Geometry: final body of the model. Coordinates: model frame, mm. Face numbers are marked on the shaded views. A direction names the side the tool comes from. Give positions to 0.01 mm unless a question says otherwise; leave off trailing zeros. Loops run counter-clockwise (first coordinate to the right, second up) from the corner with the lowest first, then second, coordinate; pieces in that order, holes last.
1. Draft query along X for the marked faces 3, 4 and 5. Return one class per face: +X half, -X half, draft (parallel to the pull), parting line (faces both ways), or undercut.
2. Section A-A, the plane y = 0. State how many separate pieces and enclosed holes the cut face has, then the cut area to 4 significant figures.
3. First-contact query: P1, Ø1.5, axis at x = 28, y = 29.5, coming from the +Z side; P2, Ø2, axis at y = -25, z = 26.5, coming from the +X side; P3, Ø1.5, axis at y = -22, z = 10.5, coming from the -X side; P4, Ø10, axis at y = -16, z = 19, coming from the -X side. Flat tips, straight axial feed; report the tip coordinate or a pass-through.
4. Material intervals for line 1 along Z through (x, y) = (29.5, 0); line 2 along Z through (x, y) = (-32, 14.5); line 3 along Y through (x, z) = (12.5, 1), sorted ascending.
5. Section D-D, the plane z = 26.5. Output: boundary loops of the cut face in (x, y).
6. Section C-C, the plane z = 5. Output: boundary loops of the cut face in (x, y), then the cut area to 3 significant figures.
7. Access query for the marked faces 1 and 2. Directions: +Z, -Z, +X, -X, +Y, -Y. A direction counts if a zero-diameter tool reaches every point of the face in a straight line with its end or side. Return the directions, or none.
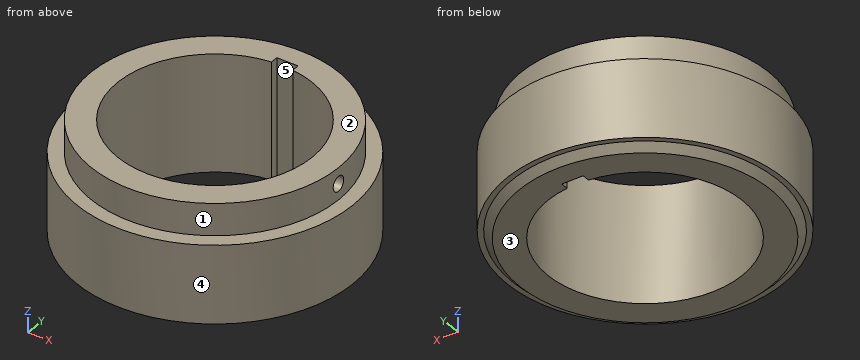
from build123d import *

# Parameters (mm, degrees)
SKETCH1_R             = 39
EXTRUDE1_DEPTH        = 22
SKETCH2_R             = 35
EXTRUDE2_DEPTH        = 9
SKETCH4_R             = 37.5
EXTRUDE4_DEPTH        = 2
EXTRUDE3_DEPTH        = 113
CHAMFER1_SIZE         = 2
M5_TAPPED_HOLE6_D     = 4.2
M5_TAPPED_HOLE6_DEPTH = 24
M5_TAPPED_HOLE6_TIP   = 1.2618073


with BuildPart() as part:
    # Sketch1 → Extrude1 (new body)
    with BuildSketch(Plane.XY):
        Circle(SKETCH1_R)
    extrude(amount=EXTRUDE1_DEPTH)

    # Sketch2 → Extrude2 (add)
    with BuildSketch(Plane.XY.offset(22)):
        Circle(SKETCH2_R)
    extrude(amount=EXTRUDE2_DEPTH)

    # Sketch4 → Extrude4 (add)
    with BuildSketch(Plane(origin=(0, 0, 0), x_dir=(-1, 0, 0), z_dir=(0, 0, -1))):
        with Locations(Location((0, 0, 0), (0, 0, 180))):
            Circle(SKETCH4_R)
    extrude(amount=EXTRUDE4_DEPTH)

    # Sketch3 → Extrude3 (cut)
    with BuildSketch(Plane.XY.offset(31)):
        with BuildLine():
            Line((-3, 29.5), (3, 29.5))
            Line((3, 29.5), (3, 27.335873866))
            ThreePointArc((3, 27.335873866), (0, -27.5), (-3, 27.335873866))
            Line((-3, 27.335873866), (-3, 29.5))
        make_face()
    extrude(amount=-EXTRUDE3_DEPTH, mode=Mode.SUBTRACT)

    # Chamfer1
    chamfer1_edges = [part.edges().sort_by_distance(p)[0] for p in [
        (-37.5, 0, -2),
    ]]
    chamfer(chamfer1_edges, length=CHAMFER1_SIZE - 0.0001)  # a hair under: the kernel refuses the full size

    # M5 Tapped Hole6
    with Locations(Plane(origin=(35, 0, 26.5), x_dir=(0, 1, 0), z_dir=(1, 0, 0))):
        with Locations((0, 0)):
            Hole(M5_TAPPED_HOLE6_D / 2, depth=M5_TAPPED_HOLE6_DEPTH)
            with Locations((0, 0, -(M5_TAPPED_HOLE6_DEPTH + M5_TAPPED_HOLE6_TIP / 2))):  # 118° drill point
                Cone(0, M5_TAPPED_HOLE6_D / 2, M5_TAPPED_HOLE6_TIP, mode=Mode.SUBTRACT)


solid = part.part
Answers below:
1. face 3: draft
1. face 4: parting line
1. face 5: undercut
2. separate pieces: 3
2. enclosed holes: 0
2. area: 645.5 mm2
3. P1: passes through
3. P2: stops at x = 25.48
3. P3: stops at x = -32.7
3. P4: stops at x = -37.42
4. line 1: z = -2 to 24.4, 28.6 to 31
4. line 2: z = -2 to 22
4. line 3: y = -36.94 to -24.49, 24.49 to 36.94
5. outline: (-3, 27.34) - (-3, 29.5) - (3, 29.5) - (3, 27.34) arc R27.5 cw to (27.42, 2.1) - (34.94, 2.1) arc R35 ccw (long way) to (34.94, -2.1) - (27.42, -2.1) arc R27.5 cw (long way) to start
6. outline: circle Ø78 at (0, 0); hole (-3, 27.34) arc R27.5 ccw (long way) to (3, 27.34) - (3, 29.5) - (-3, 29.5) - close
6. area: 2,390 mm2
7. face 1: +Z
7. face 2: +Z, +X, -X, +Y, -Y
